Geometry: final body of the model. Coordinates: model frame, mm. Face numbers are marked on the shaded views. Round coordinates to 2 decimals unless told otherwise and drop trailing zeros. Loops run counter-clockwise (first coordinate to the right, second up) from the corner with the lowest first, then second, coordinate; pieces in that order, holes last. Notation, with made-up numbers: (39.5, -23) - (56.5, -23) arc R25 ccw to (56.5, 7) - close; hole circle Ø10 at (47.5, -30). An arc over 180 degrees is marked (long way). Answer as a JSON object with one key per item and string values. Group by question number.
Item 1: Section A-A (z = 24.5). Return the cut outline in (x, y), plus the area to 3 significant figures.
Item 2: Section B-B (x = 16.6). Return the cut outline in (y, z).
Item 3: Section C-C (y = 9). Return the cut outline in (x, z).
Item 4: First-contact query: pin 1 (2 mm diameter, centred on y = 9, z = -5, fed in from -X) (3 decimals); pin 2 (1.6 mm diameter, centred on y = 2.5, z = -14, fed in from +X); pin 3 (7 mm diameter, centred on x = 13.5, y = 1.5, fed in from +Z); pin 4 (5 mm diameter, centred on y = 3, z = 24, fed in from -X). Flat tips, straight axial feed; report the tip coordinate or a pass-through.
Item 5: Section D-D (y = 3.5). Return the cut outline in (x, z), plus the area to 3 significant figures.
Item 6: Line query: line 1 (X direction, y = 5.5, z = 6.5); line 2 (Y direction, x = 0.5, z = -11.5); line 3 (Y direction, x = 24, z = -8). Output: solid intervals per line, ascending.
Item 7: Draft query along Y for the marked faces 1, 2 and 3. Return one class per face: released by +Y, released by -Y, zero draft, split by the parting line, or undercut.
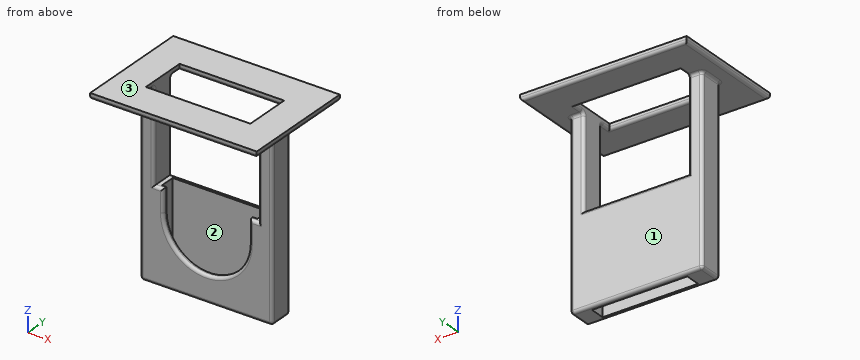
```python
from build123d import *

# Parameters (mm, degrees)
SKETCH1_W                = 36.4
SKETCH1_H                = 75.6
SKETCH1_W_2              = 33.2
SKETCH1_H_2              = 72.4
BOSS_EXTRUDE1_DEPTH      = 5.2
SKETCH2_W                = 36.4
SKETCH2_H                = 75.6
BOSS_EXTRUDE2_DEPTH      = 1.6
BOSS_EXTRUDE3_START      = 5.2
SKETCH2_2_W              = 36.4
SKETCH2_2_H              = 75.6
BOSS_EXTRUDE3_DEPTH      = 1.6
CUT_EXTRUDE1_START       = -1.6
SKETCH3_W                = 33.2
SKETCH3_H                = 1.6
CUT_EXTRUDE1_DEPTH       = 5.2
CUT_EXTRUDE2_DEPTH       = 2
SKETCH6_W                = 4.8
SKETCH6_H                = 64
BOSS_EXTRUDE5_DEPTH      = 6.8
BOSS_EXTRUDE5_DEPTH_BACK = 1.6
SKETCH7_W                = 36.4
SKETCH7_H                = 43.6
CUT_EXTRUDE3_DEPTH       = 12
SKETCH8_W                = 58
SKETCH8_H                = 40.4
SKETCH8_W_2              = 36.4
SKETCH8_H_2              = 16.4
BOSS_EXTRUDE6_DEPTH      = 2
FILLET2_R                = 1


with BuildPart() as part:
    # Sketch1 → Boss-Extrude1 (new body)
    with BuildSketch(Plane(origin=(0, 0, 0), x_dir=(1, 0, 0), z_dir=(0, 1, 0))):
        with Locations((16.6, 36.2)):
            Rectangle(SKETCH1_W, SKETCH1_H)
        with Locations((16.6, 36.2)):
            Rectangle(SKETCH1_W_2, SKETCH1_H_2, mode=Mode.SUBTRACT)
    extrude(amount=BOSS_EXTRUDE1_DEPTH)

    # Sketch2 → Boss-Extrude2 (add)
    with BuildSketch(Plane(origin=(0, 0, 0), x_dir=(1, 0, 0), z_dir=(0, 1, 0))):
        with Locations((16.6, 36.2)):
            Rectangle(SKETCH2_W, SKETCH2_H)
    extrude(amount=-BOSS_EXTRUDE2_DEPTH)

    # Sketch2_2 → Boss-Extrude3 (add)
    with BuildSketch(Plane(origin=(0, 0, 0), x_dir=(1, 0, 0), z_dir=(0, 1, 0)).offset(BOSS_EXTRUDE3_START)):
        with Locations((16.6, 36.2)):
            Rectangle(SKETCH2_2_W, SKETCH2_2_H)
    extrude(amount=BOSS_EXTRUDE3_DEPTH)

    # Sketch3 → Cut-Extrude1 (cut)
    with BuildSketch(Plane(origin=(0, 6.8, 0), x_dir=(1, 0, 0), z_dir=(0, 1, 0)).offset(CUT_EXTRUDE1_START)):
        with Locations((16.6, -0.8)):
            Rectangle(SKETCH3_W, SKETCH3_H)
    extrude(amount=-CUT_EXTRUDE1_DEPTH, mode=Mode.SUBTRACT)

    # Sketch5 → Cut-Extrude2 (cut)
    with BuildSketch(Plane.XZ.offset(1.6)):
        with BuildLine():
            Line((1.6, 1.6), (31.6, 1.6))
            Line((31.6, 1.6), (31.6, -6.4))
            ThreePointArc((31.6, -6.4), (16.6, -21.4), (1.6, -6.4))
            Line((1.6, -6.4), (1.6, 1.6))
        make_face()
    extrude(amount=-CUT_EXTRUDE2_DEPTH, mode=Mode.SUBTRACT)

    # Sketch6 → Boss-Extrude5 (add, two sides)
    with BuildSketch(Plane(origin=(0, 0, 0), x_dir=(1, 0, 0), z_dir=(0, 1, 0))) as boss_extrude5_sk:
        with Locations((-4, -1.6)):
            Rectangle(SKETCH6_W, SKETCH6_H)
        with Locations((37.2, -1.6)):
            Rectangle(SKETCH6_W, SKETCH6_H)
    extrude(amount=BOSS_EXTRUDE5_DEPTH)
    extrude(boss_extrude5_sk.sketch, amount=-BOSS_EXTRUDE5_DEPTH_BACK)

    # Sketch7 → Cut-Extrude3 (cut)
    with BuildSketch(Plane.XZ.offset(1.6)):
        with Locations((16.6, -52.2)):
            Rectangle(SKETCH7_W, SKETCH7_H)
    extrude(amount=-CUT_EXTRUDE3_DEPTH, mode=Mode.SUBTRACT)

    # Sketch8 → Boss-Extrude6 (add)
    with BuildSketch(Plane.XY.offset(33.6)):
        with Locations((16.6, 2.6)):
            Rectangle(SKETCH8_W, SKETCH8_H)
        with Locations((16.6, 2.6)):
            Rectangle(SKETCH8_W_2, SKETCH8_H_2, mode=Mode.SUBTRACT)
    extrude(amount=BOSS_EXTRUDE6_DEPTH)

    # Fillet2
    fillet2_edges = [part.edges().sort_by_distance(p)[0] for p in [
        (39.6, 2.6, -30.4),
        (39.6, -1.6, 1.6),
        (39.6, 2.6, 33.6),
        (37.2, -1.6, 33.6),
        (34.8, -1.6, 17.6),
        (34.8, 6.8, 17.6),
        (37.2, 6.8, 33.6),
        (39.6, 6.8, 1.6),
        (-1.6, -3.6, 33.6),
        (16.6, -5.6, 33.6),
        (34.8, -3.6, 33.6),
        (34.8, 8.8, 33.6),
        (16.6, 10.8, 33.6),
        (-1.6, 8.8, 33.6),
        (-12.4, 2.6, 33.6),
        (16.6, -17.6, 33.6),
        (45.6, 2.6, 33.6),
        (16.6, 22.8, 33.6),
        (0, -1.6, 1.6),
        (16.6, 6.8, 1.6),
        (33.2, -1.6, 1.6),
        (1.6, -1.6, -2.4),
        (16.6, -1.6, -21.4),
        (31.6, -1.6, -2.4),
        (-1.6, -1.6, 17.6),
        (-6.4, 2.6, -30.4),
        (16.6, -1.6, -30.4),
        (-4, -1.6, 33.6),
        (-6.4, 2.6, 33.6),
        (-6.4, -1.6, 1.6),
        (16.6, 6.8, -30.4),
        (-6.4, 6.8, 1.6),
        (-4, 6.8, 33.6),
        (-1.6, 6.8, 17.6),
    ]]
    fillet(fillet2_edges, radius=FILLET2_R)


solid = part.part
```
Values:
{
 "1": {"outline": "(-6.4, -0.6) arc R1 ccw to (-5.4, -1.6) - (-2.6, -1.6) arc R1 ccw to (-1.6, -0.6) - (-1.6, 5.8) arc R1 ccw to (-2.6, 6.8) - (-5.4, 6.8) arc R1 ccw to (-6.4, 5.8) - close; (34.8, -0.6) arc R1 ccw to (35.8, -1.6) - (38.6, -1.6) arc R1 ccw to (39.6, -0.6) - (39.6, 5.8) arc R1 ccw to (38.6, 6.8) - (35.8, 6.8) arc R1 ccw to (34.8, 5.8) - close", "area": "78.9 mm^2"},
 "2": {"outline": "(-17.6, 34.6) arc R1 ccw to (-16.6, 33.6) - (-6.6, 33.6) arc R1 ccw to (-5.6, 34.6) - (-5.6, 35.6) - (-17.6, 35.6) - close; (-1.6, -29.4) arc R1 ccw to (-0.6, -30.4) - (0, -30.4) - (0, -21.4) - (-0.6, -21.4) arc R1 ccw to (-1.6, -22.4) - close; (5.2, -30.4) - (5.8, -30.4) arc R1 ccw to (6.8, -29.4) - (6.8, 0.6) arc R1 ccw to (5.8, 1.6) - (5.2, 1.6) - close; (10.8, 34.6) arc R1 ccw to (11.8, 33.6) - (21.8, 33.6) arc R1 ccw to (22.8, 34.6) - (22.8, 35.6) - (10.8, 35.6) - close"},
 "3": {"outline": "(-12.4, 34.6) arc R1 ccw to (-11.4, 33.6) - (-2.6, 33.6) arc R1 ccw to (-1.6, 34.6) - (-1.6, 35.6) - (-12.4, 35.6) - close; (34.8, 34.6) arc R1 ccw to (35.8, 33.6) - (44.6, 33.6) arc R1 ccw to (45.6, 34.6) - (45.6, 35.6) - (34.8, 35.6) - close"},
 "4": {"pin 1": "passes through", "pin 2": "stops at x = 39.6", "pin 3": "stops at z = -20.03", "pin 4": "stops at x = -6.4"},
 "5": {"outline": "(-12.4, 34.6) arc R1 ccw to (-11.4, 33.6) - (-7.4, 33.6) arc R1 cw to (-6.4, 32.6) - (-6.4, -29.4) arc R1 ccw to (-5.4, -30.4) - (0, -30.4) - (0, 1.6) - (-1.6, 1.6) - (-1.6, 35.6) - (-12.4, 35.6) - close; (33.2, -30.4) - (38.6, -30.4) arc R1 ccw to (39.6, -29.4) - (39.6, 32.6) arc R1 cw to (40.6, 33.6) - (44.6, 33.6) arc R1 ccw to (45.6, 34.6) - (45.6, 35.6) - (34.8, 35.6) - (34.8, 1.6) - (33.2, 1.6) - close", "area": "760 mm^2"},
 "6": {"line 1": "x = -6.4 to -1.6, 34.8 to 39.6", "line 2": "y = -1.6 to 0, 5.2 to 6.8", "line 3": "y = 5.2 to 6.8"},
 "7": {"face 1": "released by +Y", "face 2": "undercut", "face 3": "zero draft"}
}
